Source: CAD feature listing. Evaluate the final solid. Frame: model axes, mm. Face numbers are marked on the shaded views. A direction names the side the tool comes from. Round coordinates to 2 decimals unless told otherwise and drop trailing zeros. Write each loop counter-clockwise with the first axis right and the second up, starting at its lowest first coordinate (ties: lowest second). Pieces come first, ordered by that corner, then holes. Notation, with made-up numbers: M 89,51.25 L 132,51.25 A14 ccw 132,67.25 Z; hole C 73.5,46 d11. An arc over 180 degrees is marked long. Answer in a Markdown table with one row per item.
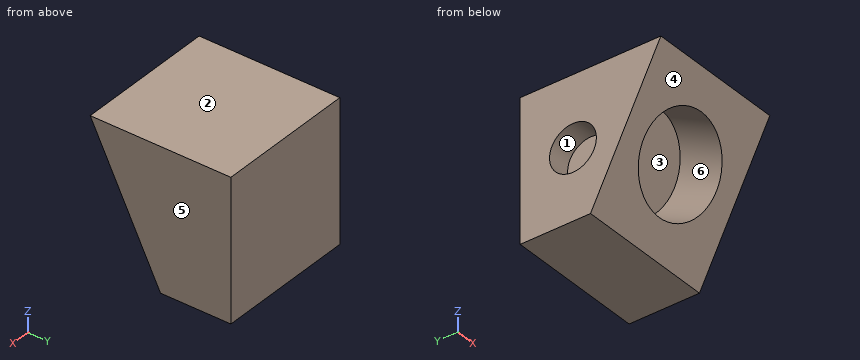
from build123d import *

# Parameters (mm, degrees)
F0_W     = 30
F0_H     = 30
F1_DEPTH = 30
F3_DEPTH = 30
F4_R     = 10
F5_DEPTH = 10
F6_R     = 5
F7_DEPTH = 5


with BuildPart() as f1:
    # F0 (on Front) → F1 (new body)
    with BuildSketch(Plane.XZ):
        Rectangle(F0_W, F0_H)
    extrude(amount=F1_DEPTH)

    # F2 (on face) → F3 (cut)
    with BuildSketch(Plane(origin=(-15, 0, 0), x_dir=(0, -1, 0), z_dir=(-1, 0, 0))):
        Polygon((30, -15), (30, 15), (15, -15), align=None)
    extrude(amount=-F3_DEPTH, mode=Mode.SUBTRACT)

    # F4 (on face) → F5 (cut)
    with BuildSketch(Plane(origin=(0, -18, -9), x_dir=(1, 0, 0), z_dir=(0, -0.894427, -0.447214))):
        with Locations((0, 10.062306)):
            Circle(F4_R)
    extrude(amount=-F5_DEPTH, mode=Mode.SUBTRACT)

    # F6 (on face) → F7 (cut)
    with BuildSketch(Plane(origin=(-15, 0, 0), x_dir=(0, -1, 0), z_dir=(-1, 0, 0))):
        with Locations((11.25, 0)):
            Circle(F6_R)
    extrude(amount=-F7_DEPTH, mode=Mode.SUBTRACT)


solid = f1.part
Q1. Section D-D (x = -2). Return loops of the section in (y, z).
Solutions:
| item | result |
|---|---|
| outline | M -30,15 L -26.88,8.76 L -17.94,13.24 L -9.17,-4.29 L -18.12,-8.76 L -15,-15 L 0,-15 L 0,15 Z |
Q2. Contact query for flat-ended pins moving along their axis: pin 1 Ø4 at (x, z) = (-6, 3) entering from -Y; pin 2 Ø2 at (x, y) = (3, -25.5) entering from -Z; pin 3 Ø12 at (x, z) = (9, 3.5) entering from -Y. Output: stop coordinate, or through.
Solutions:
| item | result |
|---|---|
| pin 1 | stops at y = -13.82 |
| pin 2 | stops at z = 8.53 |
| pin 3 | stops at y = -27.25 |
Q3. Material intervals for probe 1 along Z at (x, y) = (-12.05, -11.25); probe 2 along X at (y, z) = (-15, 4); probe 3 along Z at (x, y) = (-2.25, -15.5), sorted ascending.
Solutions:
| item | result |
|---|---|
| probe 1 | z = -15 to -5, 5 to 15 |
| probe 2 | x = -15 to -10, 10 to 15 |
| probe 3 | z = -14 to -7.39, 8.36 to 15 |
Q4. Access query for the marked faces 1, 2 and 3. Directions: +Z, -Z, +X, -X, +Y, -Y. A direction counts if a zero-diameter tool reaches every point of the face in a straight line with its end or side. Return the directions, or none.
Solutions:
| item | result |
|---|---|
| face 1 | -X |
| face 2 | +Z, +X, -X, +Y, -Y |
| face 3 | none |
Q5. Section C-C (z = -11.75). Return loops of the section in (x, y) (3 decimals), and give its area (3 significant figures).
Solutions:
| item | result |
|---|---|
| outline | M -15,-16.625 L 15,-16.625 L 15,0 L -15,0 Z |
| area | 499 mm2 |
Q6. Section A-A (x = -11.25). Return loops of the section in (y, z).
Solutions:
| item | result |
|---|---|
| outline | M -30,15 L -15,-15 L 0,-15 L 0,15 Z; hole C -11.25,0 d10 |
Q7. Pull-direction query (Y, two-part tool) for the marked faces 4, 5 and 6; classes: pulls with the +Y half, pulls with the -Y half, needs draft (parallel to the pull), parting line crosses it, or undercut.
Solutions:
| item | result |
|---|---|
| face 4 | pulls with the -Y half |
| face 5 | needs draft |
| face 6 | undercut |
Q8. Section B-B (x = 7.5). Return loops of the section in (y, z), and give its area (3 significant figures).
Solutions:
| item | result |
|---|---|
| outline | M -30,15 L -25.46,5.92 L -16.51,10.39 L -10.6,-1.44 L -19.54,-5.92 L -15,-15 L 0,-15 L 0,15 Z |
| area | 543 mm2 |
